Part model, mm, in its own coordinate system. Face numbers are marked on the shaded views. A direction names the side the tool comes from. Coordinates: 2 decimals unless noted, no trailing zeros. Loops run counter-clockwise (first coordinate to the right, second up) from the corner with the lowest first, then second, coordinate; pieces in that order, holes last. Notation, with made-up numbers: (-14.5, 54.25) - (5.5, 54.25) arc R5 cw to (5.5, 59.25) - close; hole circle Ø10 at (3, 15). An arc over 180 degrees is marked (long way). Use a Markdown table: item, result. Add a question column.
1) Probe probe 1 along Z at (x, y) = (-1.25, -1.15); probe 2 along Z at (x, y) = (0.25, 0.5) (3 decimals); probe 3 along Z at (x, y) = (0.4, 1.25). List the from-to ranges inside material, lowest first. Write a range as [from, to].
2) Tool access for the marked faces 4, 5 and 6: list every direction of +Z, -Z, +X, -X, +Y, -Y with a clear straight run to the whole face (end or side of a thin tool).
3) Band-saw the part on B-B (z = -13.5). Give the cut face in (x, y), plus the area to 3 significant figures.
4) Drop flat-ended pins along their axis: P1, Ø1.5, axis at x = 0, y = 0.5, coming from the -Z side (3 decimals); P2, Ø2, axis at x = -1, z = -12.5, coming from the -Y side; P3, Ø2, axis at x = 1.5, z = -15.5, coming from the -Y side. Give the stop position or say it passes through.
5) Band-saw the part on A-A (y = 0). Give the cut face in (x, z) (3 decimals), plus the area to 3 significant figures.
6) Pull direction Z, two halves, no side cores. Call the marked faces 1, 2 and 3: +Z half, -Z half, draft (parallel to the pull), parting line (faces both ways), or undercut.
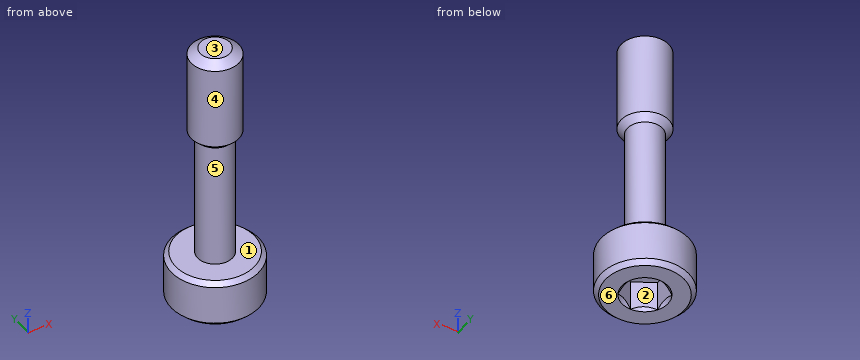
from build123d import *

# Parameters (mm, degrees)
SKETCH1_R          = 1.5
EXTRUDE1_DEPTH     = 14
SKETCH6_R          = 2.75
EXTRUDE2_DEPTH     = 3
CUT_EXTRUDE1_DEPTH = 1.875
CHAMFER1_SIZE      = 0.275
SKETCH11_OUTSIDE_W = 11.238
SKETCH11_OUTSIDE_H = 11.238
SKETCH11_OUTSIDE_R = 1.1
CUT_EXTRUDE3_DEPTH = 8


with BuildPart() as part:
    # Sketch1 → Extrude1 (new body)
    with BuildSketch(Plane.XY):
        Circle(SKETCH1_R)
    extrude(amount=-EXTRUDE1_DEPTH)

    # Sketch6 → Extrude2 (add)
    with BuildSketch(Plane(origin=(0, 0, -14), x_dir=(-1, 0, 0), z_dir=(0, 0, -1))):
        Circle(SKETCH6_R)
    extrude(amount=EXTRUDE2_DEPTH)

    # Sketch7 → Cut-Extrude1 (cut)
    with BuildSketch(Plane(origin=(0, 0, -17), x_dir=(-1, 0, 0), z_dir=(0, 0, -1))):
        Polygon((0, 1.443375673), (-1.25, 0.721687836), (-1.25, -0.721687836), (0, -1.443375673), (1.25, -0.721687836), (1.25, 0.721687836), align=None)
    extrude(amount=-CUT_EXTRUDE1_DEPTH, mode=Mode.SUBTRACT)

    # Cut-Extrude2 cone 1 section (on through the dimple's axis) → Cut-Extrude2 (revolve, cut)
    with BuildSketch(Plane(origin=(0, 0, -17), x_dir=(0, 1, 0), z_dir=(1, 0, 0))):
        Polygon((0, 0), (1.443375673, 0), (0, 1.443375673), align=None)
    revolve(axis=Axis((0, 0, -17), (0, 0, 1)), mode=Mode.SUBTRACT)

    # Chamfer1
    chamfer1_edges = [part.edges().sort_by_distance(p)[0] for p in [
        (2.75, 0, -14),
        (2.75, 0, -17),
    ]]
    chamfer(chamfer1_edges, length=CHAMFER1_SIZE)

    # Sketch11 outside → Cut-Extrude3 (cut)
    with BuildSketch(Plane.XY.offset(-14)):
        Rectangle(SKETCH11_OUTSIDE_W, SKETCH11_OUTSIDE_H)
        Circle(SKETCH11_OUTSIDE_R, mode=Mode.SUBTRACT)
    extrude(amount=CUT_EXTRUDE3_DEPTH, mode=Mode.SUBTRACT)

    # Sketch4 → Cut-Revolve1 (revolve, cut)
    with BuildSketch(Plane(origin=(0, 0, 0), x_dir=(0, 0, -1), z_dir=(1, 0, 0)), mode=Mode.PRIVATE) as cut_revolve1_sk:
        Polygon((0.405251783, 1.5), (0, 0.921240474), (0, 1.5), align=None)
        Polygon((5.6, 1.5), (6, 1.5), (6, 1.1), align=None)
    revolve(cut_revolve1_sk.sketch.rotate(Axis((0, 0, 0), (0, 0, -1)), 90), axis=Axis((0, 0, 0), (0, 0, -1)), mode=Mode.SUBTRACT)


solid = part.part
Answer block:
| question | item | result |
|---|---|---|
| 1 | probe 1 | [-17, -14] |
| 1 | probe 2 | [-15.125, 0] |
| 1 | probe 3 | [-16.87, -14], [-5.79, -0.27] |
| 2 | face 4 | +Z |
| 2 | face 5 | none |
| 2 | face 6 | -Z, +X, -X, +Y, -Y |
| 3 | outline | circle Ø2.2 at (0, 0) |
| 3 | area | 3.80 mm2 |
| 4 | P1 | z = -15.125 |
| 4 | P2 | y = -1.1 |
| 4 | P3 | y = -2.7 |
| 5 | outline | (-2.75, -16.725) - (-2.475, -17) - (-1.443, -17) - (-1.25, -16.807) - (-1.25, -15.125) - (1.25, -15.125) - (1.25, -16.807) - (1.443, -17) - (2.475, -17) - (2.75, -16.725) - (2.75, -14.275) - (2.475, -14) - (1.1, -14) - (1.1, -6) - (1.5, -5.6) - (1.5, -0.405) - (0.921, 0) - (-0.921, 0) - (-1.5, -0.405) - (-1.5, -5.6) - (-1.1, -6) - (-1.1, -14) - (-2.475, -14) - (-2.75, -14.275) - close |
| 5 | area | 46.8 mm2 |
| 6 | face 1 | undercut |
| 6 | face 2 | draft |
| 6 | face 3 | +Z half |
